Source: CAD feature listing. Evaluate the final solid. Frame: model axes, mm. Coordinates: 2 decimals unless noted, no trailing zeros. Order: outer loops, then holes, each group sorted by start corner. A loop starts at its lowest first (then second) coordinate and runs counter-clockwise, first axis right, second up.
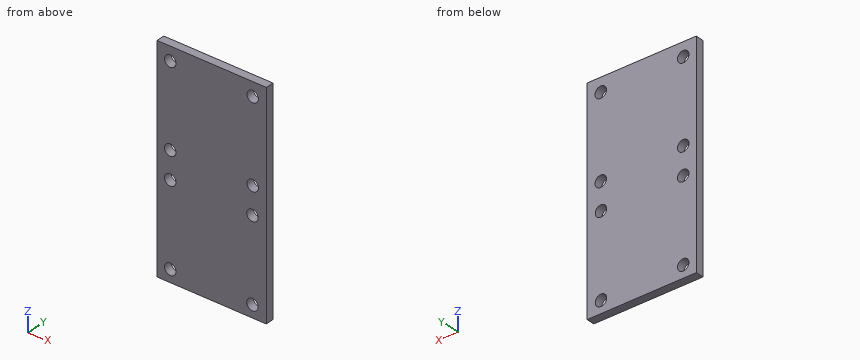
Autodesk Inventor part; units mm, degrees
ref_plane "YZ Plane" through (0, 0, 0) normal (1, 0, 0) x (0, 1, 0)
ref_plane "XZ Plane" through (0, 0, 0) normal (0, 1, 0) x (-1, 0, 0)
ref_plane "XY Plane" through (0, 0, 0) normal (0, 0, 1) x (1, 0, 0)
sketch "Sketch1" plane through (0, 0, 0) normal (0, 1, 0) x (-1, 0, 0)
  line L0 (-10, 20) -> (10, 20)
  line L1 (10, 20) -> (10, -20)
  line L2 (10, -20) -> (-10, -20)
  line L3 (-10, -20) -> (-10, 20)
  line L4 (-10, 20) -> (10, -20) construction
  line L5 (10, 20) -> (-10, -20) construction
  point P0 (0, 0)
  dimension "d0" = 40
  dimension "d1" = 20
extrude "Plate1" add sketch "Sketch1" along normal blind 1.5
sketch "Sketch2" plane through (0, 1.5, 0) normal (0, 1, 0) x (1, 0, 0)
  circle A0 centre (-7.6, -17.455) radius 0.7835
  line L0 (10, 20) -> (10, -20)
  line L1 (-10, 20) -> (10, 20)
  line L2 (-10, -20) -> (-10, 20)
  line L3 (10, -20) -> (-10, -20)
  circle A1 centre (-7.6, -2.405) radius 0.7835
  circle A2 centre (7.5, -2.405) radius 0.7835
  circle A3 centre (7.5, -17.455) radius 0.7835
  point P0 (0, 0)
sketch "Sketch3" plane through (0, 1.5, 0) normal (0, 1, 0) x (1, 0, 0)
  circle A0 centre (-7.595, 2.64) radius 0.7835
  circle A1 centre (7.455, 2.64) radius 0.7835
  circle A2 centre (-7.595, 17.74) radius 0.7835
  line L0 (10, 20) -> (10, -20)
  line L1 (-10, 20) -> (10, 20)
  line L2 (-10, -20) -> (-10, 20)
  line L3 (10, -20) -> (-10, -20)
  circle A3 centre (7.455, 17.74) radius 0.7835
  point P0 (0, 0)
hole "Hole1" at (-7.595, 1.5, -17.74) at (7.455, 1.5, -17.74) at (7.455, 1.5, -2.64) at (-7.595, 1.5, -2.64) direction (0, -1, 0) diameter 2.1 depth 1.5
hole "Hole2" at (-7.6, 1.5, 2.405) at (7.5, 1.5, 2.405) at (7.5, 1.5, 17.455) at (-7.6, 1.5, 17.455) direction (0, -1, 0) diameter 2.1 depth 1.5
equation "\"d8\" = Thickness"
equation "\"d15\" = Thickness"
equation "\"d2\" = Thickness"
equation "\"BendReliefWidth\" = Thickness"
equation "\"BendReliefDepth\" = 0.5 * Thickness"
equation "\"CornerReliefSize\" = 4 * Thickness"
equation "\"MinimumRemnant\" = 2 * Thickness"
equation "\"TransitionRadius\" = BendRadius"
equation "\"JacobiRadiusSize\" = BendRadius"
equation "\"GapSize\" = Thickness"
properties part number "axis_22_bottom_frame(middle)" material "Aluminum 6061-AHC"
1. Ray query, line 1 (X direction, y = 1.2, z = -17.74) (3 decimals); line 2 (Z direction, x = -7.6, y = 0.65) (3 decimals); line 3 (X direction, y = 1, z = 2). Return the intervals inside material, ascending.
Findings:
line 1: x = -10 to -8.645, -6.545 to 6.405, 8.505 to 10
line 2: z = -20 to -18.79, -16.69 to -3.69, -1.59 to 1.355, 3.455 to 16.405, 18.505 to 20
line 3: x = -10 to -8.57, -6.63 to 6.53, 8.47 to 10
2. Section query C-C on z = -3. Return loops of the section in (x, y).
Findings:
outline: (-10, 0) - (-8.58, 0) - (-8.58, 1.5) - (-10, 1.5) - close; (-6.61, 0) - (6.47, 0) - (6.47, 1.5) - (-6.61, 1.5) - close; (8.44, 0) - (10, 0) - (10, 1.5) - (8.44, 1.5) - close
3. Section query A-A on z = -17.74. Return loops of the section in (x, y) (3 decimals).
Findings:
outline: (-10, 0) - (-8.645, 0) - (-8.645, 1.5) - (-10, 1.5) - close; (-6.545, 0) - (6.405, 0) - (6.405, 1.5) - (-6.545, 1.5) - close; (8.505, 0) - (10, 0) - (10, 1.5) - (8.505, 1.5) - close
4. Pin query (flat end, axial travel): P1, Ø1.7, axis at x = 7.5, z = 17.455, coming from the -Y side; P2, Ø2.5, axis at x = -7.595, z = -2.64, coming from the +Y side. Return the tip coordinate at first contact, or that it passes through.
Findings:
P1: passes through
P2: stops at y = 1.5
5. Section query B-B on y = 0.35. Count the separate pieces of the cut face and the enclosed holes in it, plus the area to 3 significant figures.
Findings:
separate pieces: 1
enclosed holes: 8
area: 772 mm2
